from build123d import *

# Parameters (mm, degrees)
BOSS_EXTRUDE1_DEPTH = 22.225
BOSS_EXTRUDE2_DEPTH = 22.225
SKETCH4_W           = 28.575
SKETCH4_H           = 43.053
CUT_EXTRUDE1_DEPTH  = 125.991552151
CUT_EXTRUDE4_REACH  = 101.697
SKETCH9_W           = 28.575
SKETCH9_H           = 16.728193257
BOSS_EXTRUDE3_REACH = 142.089
SKETCH11_W          = 19.05
SKETCH11_H          = 19.05
CUT_EXTRUDE5_DEPTH  = 7.9375
BOSS_EXTRUDE6_REACH = 156.463
BOSS_EXTRUDE4_DEPTH = 3.175
CUT_EXTRUDE6_REACH  = 142.089
SKETCH19_R          = 6
CUT_EXTRUDE7_DEPTH  = 138.803544436


with BuildPart() as part:
    # Sketch1 → Boss-Extrude1 (new, symmetric)
    with BuildSketch(Plane(origin=(0, 0, 0), x_dir=(0, 0, -1), z_dir=(1, 0, 0))):
        with BuildLine():
            Line((9.525, -22.225), (9.525, 0))
            ThreePointArc((9.525, 0), (5.795727419, 7.558780899), (-2.471885813, 9.198663247))
            Line((-2.471885813, 9.198663247), (-36.703, 0))
            Line((-36.703, 0), (-36.703, -22.225))
            Line((-36.703, -22.225), (9.525, -22.225))
        make_face()
    extrude(amount=BOSS_EXTRUDE1_DEPTH, both=True)

    # Sketch3 → Boss-Extrude2 (add)
    with BuildSketch(Plane(origin=(0, 0, 0), x_dir=(-1, 0, 0), z_dir=(0, -1, 0))):
        Polygon((22.225, 9.525), (22.225, -36.703), (-22.225, -36.703), (-22.225, 9.525), (-48.940128061, 9.525), (-76.2, -17.734871939), (-76.2, -38.659838164), (-56.111331957, -93.853), (56.111331957, -93.853), (76.2, -38.659838164), (76.2, -17.734871939), (48.940128061, 9.525), align=None)
        Polygon((73.025, -19.05), (47.625, 6.35), (25.4, 6.35), (25.4, -49.403), (22.225, -49.403), (22.225, -39.878), (-22.225, -39.878), (-22.225, -49.403), (-25.4, -49.403), (-25.4, 6.35), (-47.625, 6.35), (-73.025, -19.05), (-73.025, -38.1), (-53.888173023, -90.678), (53.888173023, -90.678), (73.025, -38.1), align=None, mode=Mode.SUBTRACT)
    extrude(amount=BOSS_EXTRUDE2_DEPTH)

    # Sketch4 → Cut-Extrude1 (cut, through all)
    with BuildSketch(Plane.XZ.offset(22.225)):
        with Locations((0, 12.0015)):
            Rectangle(SKETCH4_W, SKETCH4_H)
    extrude(amount=-CUT_EXTRUDE1_DEPTH, mode=Mode.SUBTRACT)

    # Sketch6 → Cut-Revolve1 (revolve, cut)
    with BuildSketch(Plane(origin=(0, 0, 0), x_dir=(1, 0, 0), z_dir=(0, 1, 0)), mode=Mode.PRIVATE) as cut_revolve1_sk:
        Polygon((-22.225, 4), (17.775, 4), (17.775, 3), (22.225, 3), (22.225, 6.35), (78.807413882, 6.35), (78.807413882, 0), (22.225, 0), (-22.225, 0), (-88.579385408, 0), (-88.579385408, 6.35), (-22.225, 6.35), align=None)
    revolve(cut_revolve1_sk.sketch.rotate(Axis((-22.225, 0, 0), (1, 0, 0)), 180), axis=Axis((-22.225, 0, 0), (1, 0, 0)), mode=Mode.SUBTRACT)

    # Sketch9 → Cut-Extrude4 (cut, up to next)
    with BuildSketch(Plane(origin=(0, 0, 33.528), x_dir=(-1, 0, 0), z_dir=(0, 0, -1)), mode=Mode.PRIVATE) as cut_extrude4_sk1:
        with Locations((0, -7.510903372)):
            Rectangle(SKETCH9_W, SKETCH9_H)
    cut_extrude4_tool1 = extrude(cut_extrude4_sk1.sketch, amount=-CUT_EXTRUDE4_REACH, mode=Mode.PRIVATE) & part.part
    add(cut_extrude4_tool1.solids().sort_by_distance((0, -7.510903, 33.528))[0], mode=Mode.SUBTRACT)

    # Sketch10 → Boss-Extrude3 (add, up to next)
    with BuildSketch(Plane(origin=(25.4, 0, 0), x_dir=(0, 0, -1), z_dir=(1, 0, 0)), mode=Mode.PRIVATE) as boss_extrude3_sk1:
        with BuildLine():
            Line((-28.575, -17.4625), (-28.575, -12.7))
            Line((-28.575, -12.7), (-25.4, -12.7))
            Line((-25.4, -12.7), (-25.4, -22.225))
            Line((-25.4, -22.225), (-44.45, -22.225))
            Line((-44.45, -22.225), (-44.45, -12.7))
            Line((-44.45, -12.7), (-41.275, -12.7))
            Line((-41.275, -12.7), (-41.275, -17.4625))
            ThreePointArc((-41.275, -17.4625), (-34.925, -20.6375), (-28.575, -17.4625))
        make_face()
    boss_extrude3_tool1 = extrude(boss_extrude3_sk1.sketch, amount=BOSS_EXTRUDE3_REACH, mode=Mode.PRIVATE) - part.part
    boss_extrude3 = boss_extrude3_tool1.solids().sort_by_distance((25.4, -15.08125, 28.362015))[0]
    add(boss_extrude3)

    # Mirror1: Boss-Extrude3 across plane
    add(boss_extrude3.mirror(Plane(origin=(0, 0, 0), x_dir=(0, 0, 1), z_dir=(1, 0, 0))))

    # Sketch11 → Cut-Extrude5 (cut)
    with BuildSketch(Plane(origin=(0, -12.7, 0), x_dir=(1, 0, 0), z_dir=(0, 1, 0))):
        with Locations((-34.925, -25.4)):
            Rectangle(SKETCH11_W, SKETCH11_H)
        with Locations((34.925, -25.4)):
            Rectangle(SKETCH11_W, SKETCH11_H)
    extrude(amount=-CUT_EXTRUDE5_DEPTH, mode=Mode.SUBTRACT)

    # Sketch18 → Boss-Extrude6 (add, up to next)
    with BuildSketch(Plane(origin=(-44.45, 0, 0), x_dir=(0, 0, -1), z_dir=(1, 0, 0)), mode=Mode.PRIVATE) as boss_extrude6_sk1:
        with BuildLine():
            Line((-25.4, -22.225), (6.35, -22.225))
            Line((6.35, -22.225), (6.35, -19.05))
            Line((6.35, -19.05), (-4.7625, -19.05))
            Line((-4.7625, -19.05), (-4.7625, -12.7))
            ThreePointArc((-4.7625, -12.7), (-9.525, -7.9375), (-14.2875, -12.7))
            Line((-14.2875, -12.7), (-14.2875, -19.05))
            Line((-14.2875, -19.05), (-25.4, -19.05))
            Line((-25.4, -19.05), (-25.4, -22.225))
        make_face()
    boss_extrude6_tool1 = extrude(boss_extrude6_sk1.sketch, amount=-BOSS_EXTRUDE6_REACH, mode=Mode.PRIVATE) - part.part
    boss_extrude6 = boss_extrude6_tool1.solids().sort_by_distance((-44.45, -17.372872, 9.525))[0]
    add(boss_extrude6)

    # Mirror3: Boss-Extrude6 across plane
    add(boss_extrude6.mirror(Plane(origin=(0, 0, 0), x_dir=(0, 0, 1), z_dir=(1, 0, 0))))

    # Sketch14 → Cut-Revolve2 (revolve, cut)
    with BuildSketch(Plane(origin=(0, -12.7, 0), x_dir=(-1, 0, 0), z_dir=(0, -1, 0))):
        Polygon((-73.701947692, -6.0325), (-19.05, -6.0325), (-19.05, -7.14375), (-14.2875, -7.14375), (-14.2875, -9.525), (-73.701947692, -9.525), align=None)
        Polygon((14.2875, -9.525), (14.2875, -7.14375), (19.05, -7.14375), (19.05, -6.0325), (73.701947692, -6.0325), (73.701947692, -9.525), align=None)
    revolve(axis=Axis((73.701947692, -12.7, 9.525), (-1, 0, 0)), mode=Mode.SUBTRACT)

    # Sketch15 → Boss-Extrude4 (add)
    with BuildSketch(Plane(origin=(-22.225, 0, 0), x_dir=(0, 0, -1), z_dir=(1, 0, 0))):
        with BuildLine():
            Line((-39.878, -22.225), (-63.685165738, -22.225))
            Line((-63.685165738, -22.225), (-68.447876585, -15.881827396))
            ThreePointArc((-68.447876585, -15.881827396), (-60.777164568, 8.708997158), (-39.878, -6.35))
            Line((-39.878, -6.35), (-39.878, -22.225))
        make_face()
    boss_extrude4 = extrude(amount=-BOSS_EXTRUDE4_DEPTH)

    # Mirror2: Boss-Extrude4 across plane
    add(boss_extrude4.mirror(Plane(origin=(0, 0, 0), x_dir=(0, 0, 1), z_dir=(1, 0, 0))))

    # Cut-Extrude6: up to this face of the body (flat: up to its plane)
    cut_extrude6_end = Plane(part.part.faces().sort_by_distance((25.4, -9.178544074, 35.806928902))[0])
    # Sketch19 → Cut-Extrude6 (cut, up to the picked face)
    with BuildSketch(Plane.ZY.offset(25.4), mode=Mode.PRIVATE) as cut_extrude6_sk1:
        with Locations((55.753, -6.35)):
            Circle(SKETCH19_R)
    cut_extrude6_tool1 = split(extrude(cut_extrude6_sk1.sketch, amount=-CUT_EXTRUDE6_REACH, mode=Mode.PRIVATE), bisect_by=cut_extrude6_end, keep=Keep.BOTH, mode=Mode.PRIVATE)
    add(cut_extrude6_tool1.solids().sort_by(Axis((-25.4, -6.35, 55.753), (1, 0, 0)))[0], mode=Mode.SUBTRACT)

    # Sketch20 → Cut-Extrude7 (cut, through all)
    with BuildSketch(Plane.ZY.offset(22.225)):
        Polygon((3.175, -5.499261314), (-9.525, -12.831609733), (-9.525, 0), (3.175, 0), align=None)
    cut_extrude7 = extrude(amount=CUT_EXTRUDE7_DEPTH, mode=Mode.SUBTRACT)

    # Mirror4: Cut-Extrude7 across plane
    add(cut_extrude7.mirror(Plane(origin=(0, 0, 0), x_dir=(0, 0, 1), z_dir=(1, 0, 0))), mode=Mode.SUBTRACT)


solid = part.part
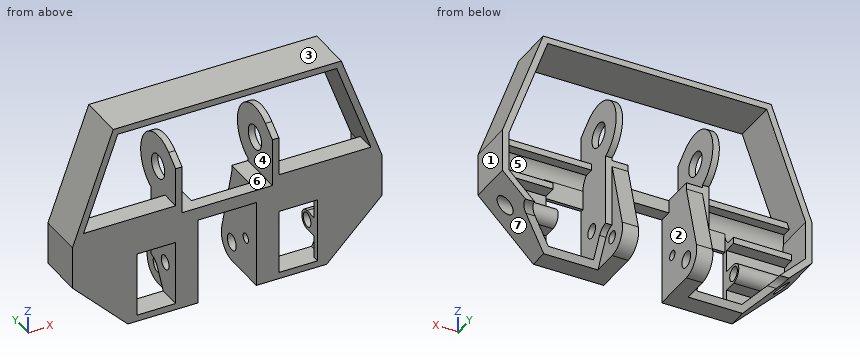
The listing builds one solid part. Answer for the finished solid, in the listing's coordinates (mm). Face numbers are marked on the shaded views. A direction names the side the tool comes from. Give positions to 0.01 mm unless a question says otherwise; leave off trailing zeros. Write each loop counter-clockwise with the first axis right and the second up, starting at its lowest first coordinate (ties: lowest second). Pieces come first, ordered by that corner, then holes.
Item 1: Find the intervals of material crossed by line 1 along Z through (x, y) = (26.5, -14) (3 decimals); line 2 along X through (y, z) = (-11, 35) (1 decimal); line 3 along X through (y, z) = (-19, 13), in increasing order.
Item 2: Section C-C, the plane y = 6.5 is taken. Write down the section's boundary in (x, z) (1 decimal), plus the area to 3 significant figures.
Item 3: Flat-ended cylindrical pins translate along their axes: P1, Ø5, axis at x = 59, z = 32.5, coming from the +Y side; P2, Ø3.5, axis at x = -48.5, z = 43.5, coming from the +Y side; P3, Ø11.5, axis at y = -13, z = 9.5, coming from the +X side. Find the tip coordinate at first contact, or state that the pin passes through.
Item 4: Section A-A, the plane x = 0 is taken. Write down the section's boundary in (y, z) (3 decimals).
Item 5: Section B-B, the plane z = 77.5 is taken. Write down the section's boundary in (x, y) (3 decimals), plus the area to 3 significant figures.
Item 6: Section D-D, the plane z = 22 is taken. Count the separate pieces of the cut face and the enclosed holes in it, plus the area to 3 significant figures.
Item 7: Which of the six approach directions +Z, -Z, +X, -X, +Y, -Y give full straight-line access (tool end or side, diameter ignored) to the marked faces 5, 6 and 7?
Item 8: Determine the mould class of the marked faces 1, 2, 3 and 4 for opening direction X: released by +X, released by -X, zero draft, split by the parting line, or undercut.
Completed:
1. line 1: z = -9.525 to -6.35, 41.275 to 44.45, 90.678 to 93.853
1. line 2: x = -76.2 to -73, -25.4 to -14.3, 14.3 to 25.4, 73 to 76.2
1. line 3: x = -71.47 to -44.45, -25.4 to -14.29, 14.29 to 25.4, 44.45 to 71.47
2. outline: (-25.4, 46.4) - (-22.2, 46.4) - (-22.2, 65.1) - (-25.4, 65.1) - close; (-22.2, -7) - (-14.3, -7) - (-14.3, 12.5) - (-22.2, 12.5) - close; (14.3, -7) - (22.2, -7) - (22.2, 12.5) - (14.3, 12.5) - close; (22.2, 46.4) - (25.4, 46.4) - (25.4, 65.1) - (22.2, 65.1) - close
2. area: 428 mm2
3. P1: stops at y = -18.92
3. P2: stops at y = -12.7
3. P3: stops at x = 73.72
4. outline: (-22.225, 33.528) - (-15.875, 33.528) - (-15.875, 39.878) - (-22.225, 39.878) - close; (-22.225, 90.678) - (0, 90.678) - (0, 93.853) - (-22.225, 93.853) - close
5. outline: (-62.063, -22.225) - (-58.685, -22.225) - (-58.685, 0) - (-62.063, 0) - close; (58.685, -22.225) - (62.063, -22.225) - (62.063, 0) - (58.685, 0) - close
5. area: 150 mm2
6. separate pieces: 4
6. enclosed holes: 0
6. area: 879 mm2
7. face 5: +Y
7. face 6: +Y, -Y
7. face 7: -Z, +X, +Y, -Y
8. face 1: released by +X
8. face 2: undercut
8. face 3: zero draft
8. face 4: undercut
